Verification items for the finished model (mm, model axes). A direction names the side the tool comes from. Give positions to 0.01 mm unless a question says otherwise; leave off trailing zeros. Loops run counter-clockwise (first coordinate to the right, second up) from the corner with the lowest first, then second, coordinate; pieces in that order, holes last. Notation, with made-up numbers: (37.25, -27) - (49.25, -27) arc R34 cw to (49.25, 12) - close; hole circle Ø1 at (66.25, 44). An arc over 180 degrees is marked (long way). One line per item, written item: value. Start each with the question number.
1. Mould release check, pull along Z, two halves, no side actions. Record for faces 1 (the cylindrical face through (-34.668, -66.054, 4.93)), 2 (the flat face through (1, -1, 0)), 3 (the cylindrical face through (0, 6, 62)): pulls with the +Z half, pulls with the -Z half, needs draft (parallel to the pull), parting line crosses it, or undercut.
2. Access from +Z, -Z, +X, -X, +Y, -Y to the whole of each face (thin tool, end or side, straight path). Record for faces 4 (the cylindrical face through (11.056, -10.138, 49.44)), 5 (the cylindrical face through (55, 0, 5)).
3. Scan lines: L1, parallel to Y at x = -32.5, z = 6; L2, parallel to X at y = -55.5, z = 6.5; L3, parallel to Z at x = 48, y = 26. Record each from-to range of solid material in increasing order. Write a range as [from, to].
4. Sectioned sample at B-B (x = 0). Record the cut outline in (y, z), plus the area to 3 significant figures.
5. Sectioned sample at D-D (y = 50). Count the separate pieces of the cut face and the enclosed holes in it, plus the area to 3 significant figures.
6. Sectioned sample at C-C (z = 75.5). Record the cut outline in (x, y), plus the area to 3 significant figures.
7. Sectioned sample at A-A (y = 0). Record the cut outline in (x, z).
from build123d import *

# Parameters (mm, degrees)
SKETCH_1_R          = 80
SKETCH_1_R_2        = 10
EXTRUDE_1_DEPTH     = 10
SKETCH_3_R          = 15
EXTRUDE_4_DEPTH     = 90
SKETCH_4_R          = 10
CUT_EXTRUDE_3_DEPTH = 45
FILLET_1_R          = 2


with BuildPart() as part:
    # 草图1 → 凸台-拉伸1 (new body)
    with BuildSketch(Plane.XY):
        Circle(SKETCH_1_R)
        with Locations((-65, 0)):
            Circle(SKETCH_1_R_2, mode=Mode.SUBTRACT)
        with Locations((-32.5, 56.291651246)):
            Circle(SKETCH_1_R_2, mode=Mode.SUBTRACT)
        with Locations((32.5, 56.291651246)):
            Circle(SKETCH_1_R_2, mode=Mode.SUBTRACT)
        with Locations((65, 0)):
            Circle(SKETCH_1_R_2, mode=Mode.SUBTRACT)
        with Locations((32.5, -56.291651246)):
            Circle(SKETCH_1_R_2, mode=Mode.SUBTRACT)
        with Locations((-32.5, -56.291651246)):
            Circle(SKETCH_1_R_2, mode=Mode.SUBTRACT)
    extrude(amount=EXTRUDE_1_DEPTH)

    # 草图3 → 凸台-拉伸4 (add)
    with BuildSketch(Plane.XY):
        with Locations(Location((0, 0, 0), (0, 0, 180))):
            Circle(SKETCH_3_R)
    extrude(amount=EXTRUDE_4_DEPTH)

    # 草图4 → 切除-拉伸3 (cut, symmetric)
    with BuildSketch(Plane(origin=(0, 0, 0), x_dir=(0, 0, -1), z_dir=(1, 0, 0))):
        with Locations(Location((-70, 0, 0), (0, 0, 180))):
            Circle(SKETCH_4_R)
    extrude(amount=CUT_EXTRUDE_3_DEPTH, both=True, mode=Mode.SUBTRACT)

    # 圆角1
    fillet_1_edges = [part.edges().sort_by_distance(p)[0] for p in [
        (-80, 0, 0),
        (-80, 0, 10),
    ]]
    fillet(fillet_1_edges, radius=FILLET_1_R)


solid = part.part
Results are:
1. face 1: needs draft
1. face 2: pulls with the -Z half
1. face 3: undercut
2. face 4: +Z
2. face 5: +Z, -Z
3. L1: y = [-73.1, -66.29], [-46.29, 46.29], [66.29, 73.1]
3. L2: x = [-57.62, -42.47], [-22.53, 22.53], [42.47, 57.62]
3. L3: z = [0, 10]
4. outline: (-80, 2) arc R2 ccw to (-78, 0) - (78, 0) arc R2 ccw to (80, 2) - (80, 8) arc R2 ccw to (78, 10) - (15, 10) - (15, 90) - (-15, 90) - (-15, 10) - (-78, 10) arc R2 ccw to (-80, 8) - close; hole circle Ø20 at (0, 70)
4. area: 3,680 mm^2
5. separate pieces: 3
5. enclosed holes: 0
5. area: 934 mm^2
6. outline: (-12.46, -8.35) arc R15 ccw to (12.46, -8.35) - close; (-12.46, 8.35) - (12.46, 8.35) arc R15 ccw to start
6. area: 233 mm^2
7. outline: (-80, 2) arc R2 ccw to (-78, 0) - (-75, 0) - (-75, 10) - (-78, 10) arc R2 ccw to (-80, 8) - close; (-55, 0) - (55, 0) - (55, 10) - (15, 10) - (15, 60) - (-15, 60) - (-15, 10) - (-55, 10) - close; (-15, 80) - (15, 80) - (15, 90) - (-15, 90) - close; (75, 0) - (78, 0) arc R2 ccw to (80, 2) - (80, 8) arc R2 ccw to (78, 10) - (75, 10) - close
